Work out the finished part from the listing and answer in its coordinate system (mm). Face numbers are marked on the shaded views. A direction names the side the tool comes from. Coordinates: 2 decimals unless noted, no trailing zeros. Order: outer loops, then holes, each group sorted by start corner. A loop starts at its lowest first (then second) coordinate and runs counter-clockwise, first axis right, second up. Notation, with made-up numbers: M 53,60 L 109,60 A23 ccw 109,82 Z; hole C 73.25,6.25 d2. An arc over 180 degrees is marked long. Use a Markdown table: item, result.
Autodesk Inventor part; units mm, degrees
ref_plane "YZ Plane" through (0, 0, 0) normal (1, 0, 0) x (0, 1, 0)
ref_plane "XZ Plane" through (0, 0, 0) normal (0, 1, 0) x (-1, 0, 0)
ref_plane "XY Plane" through (0, 0, 0) normal (0, 0, 1) x (1, 0, 0)
sketch "Sketch1" plane through (0, 0, 0) normal (0, 0, 1) x (1, 0, 0)
  line L0 (-90, 90) -> (90, 90)
  line L1 (90, 90) -> (90, -90)
  line L2 (90, -90) -> (-90, -90)
  line L3 (-90, -90) -> (-90, 90)
  line L4 (90, 40) -> (165, 40)
  line L5 (165, 40) -> (165, -40)
  line L6 (165, -40) -> (90, -40)
  line L7 (90, -40) -> (90, 40)
  point P0 (0, 0)
  point P1 (-90, 0)
  point P2 (165, 0)
  point P3 (90, 0)
  point P4 (90, -40)
  dimension "d0" = 90
  dimension "d1" = 180
  dimension "d2" = 180
  dimension "d29" = 75
  dimension "d30" = 80
extrude "Extrusion1" add sketch "Sketch1" along normal blind 10 contours L0 L1 L2 L3
sketch "Sketch3" plane through (-90, -90, 0) normal (0, -1, 0) x (1, 0, 0)
  line L0 (0, 0) -> (180, 0)
  line L1 (180, 0) -> (180, 10)
  line L2 (0, 10) -> (180, 10)
  line L3 (0, 0) -> (0, 10)
  line L4 (65, 10) -> (65, 80)
  line L5 (65, 80) -> (115, 80)
  line L6 (115, 80) -> (115, 10)
  line L7 (0, 10) -> (180, 10)
  point P0 (90, 0)
  point P1 (90, 80)
  point P2 (90, 10)
  dimension "d22" = 70
  dimension "d23" = 50
extrude "Extrusion4" add sketch "Sketch3" against normal blind 10 contours L4 L5 L6 L2
fillet "Fillet4" radius 10 6 edges at (-90, 90, 5) (90, 90, 5) (-90, -90, 5) (90, -90, 5) (-25, -85, 80) (25, -85, 80)
sketch "Sketch4" plane through (90, -40, 0) normal (0, -1, 0) x (1, 0, 0)
  line L0 (0, 0) -> (75, 0)
  line L1 (75, 0) -> (75, 10)
  line L2 (0, 10) -> (75, 10)
  line L3 (0, 0) -> (0, 10)
  line L4 (75, 10) -> (62.895, 55.1764)
  arc A0 (62.895, 55.1764) -> (27.3654, 61.7133) centre (43.5765, 50) ccw
  line L5 (0, 10) -> (-10, 10)
  line L6 (-10, 10) -> (27.3654, 61.7133)
  point P0 (-90, 0)
  dimension "d31" = 75
  dimension "d32" = 20
  dimension "d33" = 40
  dimension "d36" = 10
equation "\"d24\" = d3"
properties part number "PWTR-0082" material "Aluminum 6061"
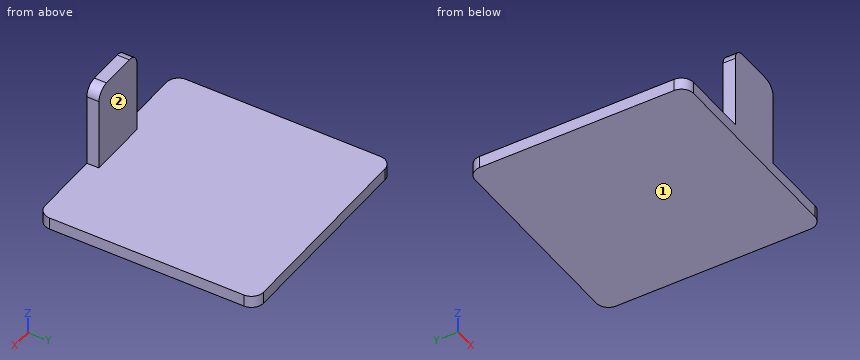
(1) Straight lines are drawn through the part: L1, parallel to Z at x = -79, y = 64; L2, parallel to Y at x = -0.5, z = 45. For each, find the intervals that lie inside material, in ascending order.
Conclusion:
| item | result |
|---|---|
| L1 | 0 to 10 |
| L2 | -90 to -80 |
(2) A cutting plane is placed at D-D (x = -7.5). Determine the outline of the cut face in (y, z).
Conclusion:
| item | result |
|---|---|
| outline | M -90,0 L 90,0 L 90,10 L -80,10 L -80,80 L -90,80 Z |
(3) Given P1, Ø15, axis at x = -7.5, z = 50, coming from the +Y side; P2, Ø5, axis at y = -84.5, z = 29.5, coming from the +X side; P3, Ø1, axis at x = 63.5, y = 55.5, coming from the +Z side, each flat-ended and moving along its own axis, determine where each tip first touches the part or whether it passes through.
Conclusion:
| item | result |
|---|---|
| P1 | y = -80 |
| P2 | x = 25 |
| P3 | z = 10 |
(4) Which of the six approach directions +Z, -Z, +X, -X, +Y, -Y give full straight-line access (tool end or side, diameter ignored) to the marked faces 1 and 2?
Conclusion:
| item | result |
|---|---|
| face 1 | -Z, +X, -X, +Y, -Y |
| face 2 | +Z, +X, -X, +Y |
(5) A cutting plane is placed at B-B (z = 44). Determine the outline of the cut face in (x, y).
Conclusion:
| item | result |
|---|---|
| outline | M -25,-90 L 25,-90 L 25,-80 L -25,-80 Z |
(6) A cutting plane is placed at C-C (y = 19.5). Determine the outline of the cut face in (x, z), then the cut area to 3 significant figures.
Conclusion:
| item | result |
|---|---|
| outline | M -90,0 L 90,0 L 90,10 L -90,10 Z |
| area | 1,800 mm2 |
(7) A cutting plane is placed at A-A (x = 21). Determine the outline of the cut face in (y, z).
Conclusion:
| item | result |
|---|---|
| outline | M -90,0 L 90,0 L 90,10 L -80,10 L -80,78 L -90,78 Z |
